```python
from build123d import *

# Parameters (mm, degrees)
EXTRUDE_5_DEPTH     = 65
SHELL_START         = -21.613486842
SHELL_8_OUTLINE_W   = 115
SHELL_8_OUTLINE_H   = 60
SHELL_8_DEPTH       = 60
SKETCH_7_W          = 18.544828657
SKETCH_7_H          = 32.414144312
CUT_EXTRUDE_1_DEPTH = 10
SKETCH_8_W          = 18.115550217
SKETCH_8_H          = 32.585855688
CUT_EXTRUDE_2_DEPTH = 10
SKETCH_9_W          = 63.329623263
SKETCH_9_H          = 52.442260972
CUT_EXTRUDE_3_DEPTH = 5
SKETCH_10_W         = 13.132979269
SKETCH_10_H         = 35.444448456
CUT_EXTRUDE_4_DEPTH = 15
SKETCH_11_W         = 60
SKETCH_11_H         = 20.052739579
CUT_EXTRUDE_5_DEPTH = 5
SKETCH_12_W         = 24.640582522
SKETCH_12_H         = 9.272414329
CUT_EXTRUDE_6_DEPTH = 5


# Read off the part's stored shape, not the designer's step: 抽壳8
with BuildPart() as part:
    # 草图1<7> → 凸台-拉伸5 (new body)
    with BuildSketch(Plane(origin=(0, 0, 0), x_dir=(1, 0, 0), z_dir=(0, 1, 0))):
        with BuildLine():
            Line((-41.756578947, 26.613486842), (73.243421053, 26.613486842))
            ThreePointArc((73.243421053, 26.613486842), (76.778954959, 25.149020748), (78.243421053, 21.613486842))
            Line((78.243421053, 21.613486842), (78.243421053, -38.386513158))
            ThreePointArc((78.243421053, -38.386513158), (76.778954959, -41.922047064), (73.243421053, -43.386513158))
            Line((73.243421053, -43.386513158), (-41.756578947, -43.386513158))
            ThreePointArc((-41.756578947, -43.386513158), (-45.292112853, -41.922047064), (-46.756578947, -38.386513158))
            Line((-46.756578947, -38.386513158), (-46.756578947, 21.613486842))
            ThreePointArc((-46.756578947, 21.613486842), (-45.292112853, 25.149020748), (-41.756578947, 26.613486842))
        make_face()
    extrude(amount=EXTRUDE_5_DEPTH)

    # 抽壳8 outline → 抽壳8 (cut)
    with BuildSketch(Plane.XY.offset(SHELL_START)):
        with Locations((15.743421053, 30)):
            Rectangle(SHELL_8_OUTLINE_W, SHELL_8_OUTLINE_H)
    extrude(amount=SHELL_8_DEPTH, mode=Mode.SUBTRACT)

    # 草图7 → 切除-拉伸1 (cut)
    with BuildSketch(Plane.XY.offset(43.386513158)):
        with Locations((25.015835382, 16.207072156)):
            Rectangle(SKETCH_7_W, SKETCH_7_H)
    extrude(amount=-CUT_EXTRUDE_1_DEPTH, mode=Mode.SUBTRACT)

    # 草图8 → 切除-拉伸2 (cut)
    with BuildSketch(Plane.XY.offset(43.386513158)):
        with Locations((3.337274103, 48.707072156)):
            Rectangle(SKETCH_8_W, SKETCH_8_H)
    extrude(amount=-CUT_EXTRUDE_2_DEPTH, mode=Mode.SUBTRACT)

    # 草图9 → 切除-拉伸3 (cut)
    with BuildSketch(Plane(origin=(0, 0, -26.613486842), x_dir=(-1, 0, 0), z_dir=(0, 0, -1))):
        with Locations((-15.743421053, 65)):
            Rectangle(SKETCH_9_W, SKETCH_9_H)
    extrude(amount=-CUT_EXTRUDE_3_DEPTH, mode=Mode.SUBTRACT)

    # 草图10 → 切除-拉伸4 (cut)
    with BuildSketch(Plane(origin=(0, 0, -26.613486842), x_dir=(-1, 0, 0), z_dir=(0, 0, -1))):
        with Locations((-71.676931419, 34.167210529)):
            Rectangle(SKETCH_10_W, SKETCH_10_H)
    extrude(amount=-CUT_EXTRUDE_4_DEPTH, mode=Mode.SUBTRACT)

    # 草图11 → 切除-拉伸5 (cut)
    with BuildSketch(Plane.ZY.offset(46.756578947)):
        with Locations((8.386513158, 29.654328955)):
            Rectangle(SKETCH_11_W, SKETCH_11_H)
    extrude(amount=-CUT_EXTRUDE_5_DEPTH, mode=Mode.SUBTRACT)

    # 草图12 → 切除-拉伸6 (cut)
    with BuildSketch(Plane(origin=(0, 65, 0), x_dir=(1, 0, 0), z_dir=(0, 1, 0))):
        with Locations((51.158892447, -28.906022645)):
            Rectangle(SKETCH_12_W, SKETCH_12_H)
    extrude(amount=-CUT_EXTRUDE_6_DEPTH, mode=Mode.SUBTRACT)


solid = part.part
```
For this review, take the finished solid that the model builds, in its own axes (mm). A direction names the side the tool comes from. Round coordinates to 2 decimals unless told otherwise and drop trailing zeros. Write each loop counter-clockwise with the first axis right and the second up, starting at its lowest first coordinate (ties: lowest second). Pieces come first, ordered by that corner, then holes.
1) Take a section at D-D on x = 49.5. Give the boundary of the cut face in (y, z).
Answer below:
outline: (0, -26.61) - (65, -26.61) - (65, 24.27) - (60, 24.27) - (60, -21.61) - (0, -21.61) - close; (0, 38.39) - (60, 38.39) - (60, 33.54) - (65, 33.54) - (65, 43.39) - (0, 43.39) - close
2) Take a section at C-C on x = 10.5. Give the boundary of the cut face in (y, z), then the cut area to 3 significant figures.
Answer below:
outline: (0, -26.61) - (38.78, -26.61) - (38.78, -21.61) - (0, -21.61) - close; (0, 38.39) - (32.41, 38.39) - (32.41, 43.39) - (0, 43.39) - close; (60, -21.61) - (65, -21.61) - (65, 33.39) - (60, 33.39) - close
area: 631 mm2
3) For line 1 along Z through (x, y) = (-31, 54.5); line 2 along X through (y, z) = (7.5, -10); line 3 along Y through (x, z) = (73, 15), list the stretches that pass through material, from the lowest coordinate up.
Answer below:
line 1: z = -26.61 to -21.61, 38.39 to 43.39
line 2: x = -46.76 to -41.76, 73.24 to 78.24
line 3: y = 60 to 65
4) Take a section at A-A on z = 19. Give the boundary of the cut face in (x, y), then the cut area to 3 significant figures.
Answer below:
outline: (-46.76, 0) - (-41.76, 0) - (-41.76, 19.63) - (-46.76, 19.63) - close; (-46.76, 39.68) - (-41.76, 39.68) - (-41.76, 60) - (73.24, 60) - (73.24, 0) - (78.24, 0) - (78.24, 65) - (-46.76, 65) - close
area: 1,120 mm2
5) Insertion check: pin 1 Ø5.5 at (x, y) = (12, 61.5) entering from -Z; pin 2 Ø1.5 at (y, z) = (24, 41) entering from +X; pin 3 Ø10 at (x, y) = (-15.5, 53) entering from -Z; pin 4 Ø1.5 at (y, z) = (48, -23.5) entering from +X. Each pin has a flat end and moves straight along its axis. Give the tip position at first contact, or say it passes through.
Answer below:
pin 1: stops at z = -21.61
pin 2: stops at x = 77.88
pin 3: stops at z = -26.61
pin 4: stops at x = 65.11
6) Machinability: for faces 1 (the face through (75, 51.889, -21)), 2 (the face through (15.743, 16, 41)), 3 (the face through (51, 63, 33.542)), which of the approach directions +Z, -Z, +X, -X, +Y, -Y give a long, thin tool a straight path to every point of the face, cutting with its end or side? Answer none if there is none.
Answer below:
face 1: -Z, +X
face 2: +Z, -Y
face 3: +Y, -Y
7) Take a section at B-B on y = 58.5. Give the boundary of the cut face in (x, z).
Answer below:
outline: (-46.76, -21.61) arc R5 ccw to (-41.76, -26.61) - (-15.92, -26.61) - (-15.92, -21.61) - (-41.76, -21.61) - (-41.76, 38.39) - (-5.72, 38.39) - (-5.72, 43.39) - (-41.76, 43.39) arc R5 ccw to (-46.76, 38.39) - close; (12.4, 38.39) - (73.24, 38.39) - (73.24, -21.61) - (47.41, -21.61) - (47.41, -26.61) - (73.24, -26.61) arc R5 ccw to (78.24, -21.61) - (78.24, 38.39) arc R5 ccw to (73.24, 43.39) - (12.4, 43.39) - close
8) Mouldability with a two-part tool opening along Z and no side actions: class faces 4 (the face through (51, 63, 24.27)), 5 (the face through (-45.253, 32.045, 41.961)), 6 (the face through (17, 65, 8)), 7 (the face through (76, 34, -11.613)) as +Z half, -Z half, draft (parallel to the pull), parting line (faces both ways), or undercut.
Answer below:
face 4: undercut
face 5: +Z half
face 6: draft
face 7: -Z half
